from build123d import *

# Parameters (mm, degrees)
F0_W     = 139.7
F0_H     = 101.6
F1_DEPTH = 6.35
F2_W     = 76.2
F2_H     = 6.35
F3_DEPTH = 6.35
F4_W     = 6.35
F4_H     = 50.8
F5_DEPTH = 6.35


with BuildPart() as f1:
    # F0 (on Front) → F1 (new body)
    with BuildSketch(Plane.XZ):
        with Locations((0, 50.8)):
            Rectangle(F0_W, F0_H)
    extrude(amount=F1_DEPTH)

    # F2 (on face) → F3 (join)
    with BuildSketch(Plane.XZ.offset(6.35)):
        with Locations((0, -3.175)):
            Rectangle(F2_W, F2_H)
    extrude(amount=-F3_DEPTH)

    # F4 (on face) → F5 (join)
    with BuildSketch(Plane.XZ.offset(6.35)):
        with Locations((-73.025, 50.8)):
            Rectangle(F4_W, F4_H)
        with Locations((73.025, 50.8)):
            Rectangle(F4_W, F4_H)
    extrude(amount=-F5_DEPTH)


solid = f1.part
Model file for the job. Use its own axes, mm. A direction names the side the tool comes from. Round coordinates to 2 decimals unless told otherwise and drop trailing zeros. Order: outer loops, then holes, each group sorted by start corner. A loop starts at its lowest first (then second) coordinate and runs counter-clockwise, first axis right, second up.
(1) Band-saw the part on A-A (y = -2.5). List the corners of the cut face in (x, z), then the cut area to 3 significant figures.
(2) Pin check, flat tips, straight feed: pin 1 (1.5 mm diameter, centred on y = -4.5, z = 80, fed in from -X); pin 2 (1.9 mm diameter, centred on x = 57.5, y = -4, fed in from -Z); pin 3 (3 mm diameter, centred on y = -2.5, z = 15, fed in from +X). Stop position of each tip, or through.
(3) Drill centre lines: line 1 (X direction, y = -1.5, z = 96); line 2 (Z direction, x = -63.5, y = -4). Where is each one in solid material? Low to high.
(4) Band-saw the part on C-C (z = 80). List the corners of the cut face in (x, y), then the cut area to 3 significant figures.
(5) 3-axis set-ups, long thin cutter, end or side, ignore diameter. For faces 1 (the face through (-38.1, -3, -3)), 2 (the face through (73, -3, 76.2)), 3 (the face through (54, -3, 0)), 4 (the face through (-73, -3, 76.2)): which of +Z, -Z, +X, -X, +Y, -Y reach the whole face in a straight line?
(6) Band-saw the part on B-B (x = -40). List the corners of the cut face in (y, z).
Verdict:
1. outline: (-76.2, 25.4) - (-69.85, 25.4) - (-69.85, 0) - (-38.1, 0) - (-38.1, -6.35) - (38.1, -6.35) - (38.1, 0) - (69.85, 0) - (69.85, 25.4) - (76.2, 25.4) - (76.2, 76.2) - (69.85, 76.2) - (69.85, 101.6) - (-69.85, 101.6) - (-69.85, 76.2) - (-76.2, 76.2) - close
1. area: 15,300 mm2
2. pin 1: stops at x = -69.85
2. pin 2: stops at z = 0
2. pin 3: stops at x = 69.85
3. line 1: x = -69.85 to 69.85
3. line 2: z = 0 to 101.6
4. outline: (-69.85, -6.35) - (69.85, -6.35) - (69.85, 0) - (-69.85, 0) - close
4. area: 887 mm2
5. face 1: -Z, -X, +Y, -Y
5. face 2: +Z, +X, +Y, -Y
5. face 3: -Z, +X, +Y, -Y
5. face 4: +Z, -X, +Y, -Y
6. outline: (-6.35, 0) - (0, 0) - (0, 101.6) - (-6.35, 101.6) - close
